Autodesk Inventor part; units mm, degrees
ref_plane "YZ Plane" through (0, 0, 0) normal (1, 0, 0) x (0, 1, 0)
ref_plane "XZ Plane" through (0, 0, 0) normal (0, 1, 0) x (-1, 0, 0)
ref_plane "XY Plane" through (0, 0, 0) normal (0, 0, 1) x (1, 0, 0)
sketch "Sketch1" plane through (0, 0, 0) normal (0, 1, 0) x (-1, 0, 0)
  line L0 (170, 50) -> (-170, 50)
  line L1 (-170, 50) -> (-170, -50)
  line L2 (-170, -50) -> (170, -50)
  line L3 (170, -50) -> (170, 50)
  line L4 (170, 50) -> (-170, -50) construction
  line L5 (-170, 50) -> (170, -50) construction
  point P0 (0, 0)
  dimension "d0" = 340
  dimension "d1" = 100
extrude "Extrusion1" add sketch "Sketch1" along normal blind 1.5875
sketch "Sketch2" plane through (0, 1.5875, 0) normal (0, 1, 0) x (1, 0, 0)
  line L0 (-170, -50) -> (170, -50)
  line L1 (170, -50) -> (170, 50)
  line L2 (170, 50) -> (-170, 50)
  line L3 (-170, 50) -> (-170, -50)
  point P0 (0, 0)
  point P1 (-160, -40)
  dimension "d4" = 10
  dimension "d5" = 10
hole "Hole1" at (-160, 1.5875, 40) direction (0, -1, 0) diameter 5.5 end through all
pattern_linear "Rectangular Pattern1" count 2 spacing 80 along (0, 0, -1) count 5 spacing 80 along (1, 0, 0) of "Hole1"
equation "\"d1\" = depth"
equation "\"d2\" = facingGasketThickness"
equation "\"mppcMountThickness\" = 6.35"
equation "\"depth\" = 100"
equation "\"facingThickness\" = 12.7"
equation "\"facingGasketThickness\" = 1.5875"
properties part number "sideGasket" material "Rubber"
Geometry: final body of the model. Coordinates: model frame, mm. Coordinates: 2 decimals unless noted, no trailing zeros. Answer in a Markdown table with one row per item.
Item 1: Ray query, L1, parallel to X at y = 0.8, z = -40; L2, parallel to Z at x = 160, y = 0.45; L3, parallel to X at y = 0.6, z = 42. Return the intervals inside material, ascending.
Return value:
| item | result |
|---|---|
| L1 | x = -170 to -162.75, -157.25 to -82.75, -77.25 to -2.75, 2.75 to 77.25, 82.75 to 157.25, 162.75 to 170 |
| L2 | z = -50 to -42.75, -37.25 to 37.25, 42.75 to 50 |
| L3 | x = -170 to -161.89, -158.11 to -81.89, -78.11 to -1.89, 1.89 to 78.11, 81.89 to 158.11, 161.89 to 170 |
Item 2: Draft query along Z for faces 1 (the cylindrical face through (-158.327, 0.783, 37.818)), 2 (the flat face through (2, 0, 1)). Return one class per face: released by +Z, released by -Z, zero draft, split by the parting line, or undercut.
Return value:
| item | result |
|---|---|
| face 1 | undercut |
| face 2 | zero draft |
Item 3: Contact query for a flat-ended pin moving along its axis: P1, Ø3.5, axis at x = 0, z = 40, coming from the -Y side. Output: stop coordinate, or through.
Return value:
| item | result |
|---|---|
| P1 | passes through |
